Geometry: final body of the model. Coordinates: model frame, mm. A direction names the side the tool comes from. Give positions to 0.01 mm unless a question says otherwise; leave off trailing zeros. Loops run counter-clockwise (first coordinate to the right, second up) from the corner with the lowest first, then second, coordinate; pieces in that order, holes last.
```python
from build123d import *

# Parameters (mm, degrees)
SKETCH_1_W          = 6
SKETCH_1_H          = 6
EXTRUDE_1_DEPTH     = 0.5
SKETCH_2_W          = 6
SKETCH_2_H          = 6
SKETCH_2_W_2        = 5.2
SKETCH_2_H_2        = 5.2
EXTRUDE_2_DEPTH     = 2
SKETCH_3_W          = 5.2
SKETCH_3_H          = 1.8
CUT_EXTRUDE_1_DEPTH = 8
SKETCH_4_W          = 5.2
SKETCH_4_H          = 1.8
CUT_EXTRUDE_2_DEPTH = 8
SKETCH_5_R          = 0.5
EXTRUDE_3_DEPTH     = 0.6
SKETCH_6_W          = 5.2
SKETCH_6_H          = 0.4
EXTRUDE_4_DEPTH     = 0.5
SKETCH_7_W          = 0.4
SKETCH_7_H          = 5.2
EXTRUDE_5_DEPTH     = 0.5
SKETCH_8_W          = 0.4
SKETCH_8_H          = 5.2
EXTRUDE_6_DEPTH     = 1
SKETCH_9_W          = 5.2
SKETCH_9_H          = 0.4
EXTRUDE_7_DEPTH     = 1
SKETCH_10_W         = 0.4
SKETCH_10_H         = 1
SKETCH_10_W_2       = 1
SKETCH_10_H_2       = 0.4
CUT_EXTRUDE_3_DEPTH = 0.5
FILLET_2_R          = 0.4


with BuildPart() as part:
    # 草图1 → 凸台-拉伸1 (new body)
    with BuildSketch(Plane(origin=(0, 0, 0), x_dir=(1, 0, 0), z_dir=(0, 1, 0))):
        Rectangle(SKETCH_1_W, SKETCH_1_H)
    extrude(amount=EXTRUDE_1_DEPTH)

    # 草图2 → 凸台-拉伸2 (add)
    with BuildSketch(Plane.XZ):
        Rectangle(SKETCH_2_W, SKETCH_2_H)
        Rectangle(SKETCH_2_W_2, SKETCH_2_H_2, mode=Mode.SUBTRACT)
    extrude(amount=EXTRUDE_2_DEPTH)

    # 草图3 → 切除-拉伸1 (cut, through all)
    with BuildSketch(Plane.ZY.offset(3)):
        with Locations((0, -1.1)):
            Rectangle(SKETCH_3_W, SKETCH_3_H)
    extrude(amount=-CUT_EXTRUDE_1_DEPTH, mode=Mode.SUBTRACT)

    # 草图4 → 切除-拉伸2 (cut, through all)
    with BuildSketch(Plane(origin=(0, 0, -3), x_dir=(-1, 0, 0), z_dir=(0, 0, -1))):
        with Locations((0, -1.1)):
            Rectangle(SKETCH_4_W, SKETCH_4_H)
    extrude(amount=-CUT_EXTRUDE_2_DEPTH, mode=Mode.SUBTRACT)

    # 草图5 → 凸台-拉伸3 (add)
    with BuildSketch(Plane.XZ.offset(2)):
        with BuildLine():
            Line((3, 2.6), (3.6, 2.6))
            ThreePointArc((3.6, 2.6), (4.307106781, 4.307106781), (2.6, 3.6))
            Line((2.6, 3.6), (2.6, 3))
            Line((2.6, 3), (3, 3))
            Line((3, 3), (3, 2.6))
        make_face()
        with Locations(Location((3.6, 3.6, 0), (0, 0, 270))):
            Circle(SKETCH_5_R, mode=Mode.SUBTRACT)
    extrude(amount=-EXTRUDE_3_DEPTH)

    # 草图6 → 凸台-拉伸4 (add)
    with BuildSketch(Plane.XZ.offset(0.2)):
        with Locations((0, 2.8)):
            Rectangle(SKETCH_6_W, SKETCH_6_H)
    extrude(amount=EXTRUDE_4_DEPTH)

    # 草图7 → 凸台-拉伸5 (add)
    with BuildSketch(Plane.XZ.offset(0.2)):
        with Locations((2.8, 0)):
            Rectangle(SKETCH_7_W, SKETCH_7_H)
    extrude(amount=EXTRUDE_5_DEPTH)

    # 草图8 → 凸台-拉伸6 (add)
    with BuildSketch(Plane.XZ.offset(0.2)):
        with Locations((-2.8, 0)):
            Rectangle(SKETCH_8_W, SKETCH_8_H)
    extrude(amount=EXTRUDE_6_DEPTH)

    # 草图9 → 凸台-拉伸7 (add)
    with BuildSketch(Plane.XZ.offset(0.2)):
        with Locations((0, -2.8)):
            Rectangle(SKETCH_9_W, SKETCH_9_H)
    extrude(amount=EXTRUDE_7_DEPTH)

    # 草图10 → 切除-拉伸3 (cut)
    with BuildSketch(Plane.XZ.offset(1.2)):
        with Locations((-2.8, 0)):
            Rectangle(SKETCH_10_W, SKETCH_10_H)
        with Locations((0, -2.8)):
            Rectangle(SKETCH_10_W_2, SKETCH_10_H_2)
    extrude(amount=-CUT_EXTRUDE_3_DEPTH, mode=Mode.SUBTRACT)

    # 圆角2
    fillet_2_edges = [part.edges().sort_by_distance(p)[0] for p in [
        (-3, -0.75, -3),
    ]]
    fillet(fillet_2_edges, radius=FILLET_2_R)


solid = part.part
```
Q1. Section query C-C, the plane x = 1.25. Return loops of the section in (y, z), and give its area (3 significant figures).
Q2. Reachability of faces 1 (the face through (0, 0, 0)), 2 (the face through (2.6, -1.5, 2.87)), 3 (the face through (-3, 0, 0)) from +Z, -Z, +X, -X, +Y, -Y: full face, straight path, thin tool, end or side. Return the list, or none.
Q3. Section query B-B, the plane y = -0.25. Return loops of the section in (x, z).
Q4. Mould query, pull axis Z, two halves, no side actions, for faces 4 (the face through (0, 0.5, 0)), 5 (the face through (2.87, -1.49, 2.6)), 6 (the face through (0, 0, 3)). Classes: +Z half, -Z half, draft (parallel to the pull), parting line (faces both ways), or undercut.
Q5. Pin query (flat end, axial travel): pin 1 Ø1.2 at (x, y) = (-0.5, -0.5) entering from +Z; pin 2 Ø0.8 at (x, y) = (3.5, -1.5) entering from -Z; pin 3 Ø0.8 at (y, z) = (0, 1) entering from +X. Return the tip coordinate at first contact, or that it passes through.
Q6. Material intervals for probe 1 along X at (y, z) = (-1.65, 3.6); probe 2 along Y at (x, z) = (0.25, -2.5); probe 3 along Z at (x, y) = (0.25, -0.4), sorted ascending.
Q7. Section query A-A, the plane y = -1.5. Return loops of the section in (x, z), and give its area (3 significant figures).
Q8. Section query D-D, the plane z = 0.25. Return loops of the section in (x, y), and give its area (3 significant figures).
Resolved:
1. outline: (-1.2, -3) - (0.5, -3) - (0.5, 3) - (-0.7, 3) - (-0.7, 2.6) - (0, 2.6) - (0, -2.6) - (-1.2, -2.6) - close
1. area: 3.76 mm2
2. face 1: -Y
2. face 2: +Z, -Y
2. face 3: +Z, -Z, -X, +Y, -Y
3. outline: (-3, -2.6) arc R0.4 ccw to (-2.6, -3) - (3, -3) - (3, 3) - (-3, 3) - close; hole (-2.6, -2.6) - (2.6, -2.6) - (2.6, 2.6) - (-2.6, 2.6) - close
4. face 4: draft
4. face 5: undercut
4. face 6: +Z half
5. pin 1: stops at z = 3
5. pin 2: stops at z = 2.6
5. pin 3: stops at x = 3
6. probe 1: x = 2.6 to 3.1, 4.1 to 4.6
6. probe 2: y = 0 to 0.5
6. probe 3: z = -3 to -2.6, 2.6 to 3
7. outline: (-3, -2.6) arc R0.4 ccw to (-2.6, -3) - (-2.6, -2.6) - close; (-3, 2.6) - (-2.6, 2.6) - (-2.6, 3) - (-3, 3) - close; (2.6, -3) - (3, -3) - (3, -2.6) - (2.6, -2.6) - close; (2.6, 2.6) - (3.6, 2.6) arc R1 ccw (long way) to (2.6, 3.6) - close; hole circle Ø1 at (3.6, 3.6)
7. area: 3.02 mm2
8. outline: (-3, -0.7) - (-2.6, -0.7) - (-2.6, 0) - (2.6, 0) - (2.6, -0.7) - (3, -0.7) - (3, 0.5) - (-3, 0.5) - close
8. area: 3.56 mm2
